```python
from build123d import *

# Parameters (mm, degrees)
BOSS_EXTRUDE1_DEPTH = 16
FILLET1_R           = 2
SKETCH2_W           = 15
SKETCH2_H           = 4.5
SKETCH2_H_2         = 6
SKETCH2_R           = 0.75
CUT_EXTRUDE1_DEPTH  = 32
SKETCH4_R           = 1.6
CUT_EXTRUDE2_DEPTH  = 92
CUT_EXTRUDE4_DEPTH  = 80.584099309
BOSS_EXTRUDE2_DEPTH = 3
DRAFT1_ANGLE        = 70
DRAFT2_START        = -8.5
DRAFT2_DEPTH        = 3
CUT_EXTRUDE5_DEPTH  = 0.5
FILLET4_R           = 0.5
FILLET3_R           = 2
CHAMFER1_SIZE       = 3


# Read off the part's stored shape, not the designer's step: Draft2
with BuildPart() as part:
    # Sketch1 → Boss-Extrude1 (new, symmetric)
    with BuildSketch(Plane(origin=(0, 0, 0), x_dir=(0, 0, -1), z_dir=(1, 0, 0))):
        Polygon((0, 16), (0, -17), (25.401923789, -60.997422612), (47.052558883, -48.497422612), (45.552558883, -45.899346401), (26.5, -56.899346401), (3, -16.196152423), (3, 16), align=None)
    extrude(amount=BOSS_EXTRUDE1_DEPTH, both=True)

    # Fillet1
    fillet1_edges = [part.edges().sort_by_distance(p)[0] for p in [
        (-16, 16, -1.5),
        (16, 16, -1.5),
    ]]
    fillet(fillet1_edges, radius=FILLET1_R)

    # Sketch2 → Cut-Extrude1 (cut)
    with BuildSketch(Plane(origin=(0, 0, -3), x_dir=(-1, 0, 0), z_dir=(0, 0, -1))):
        with Locations((0, 5.25)):
            Rectangle(SKETCH2_W, SKETCH2_H)
        Rectangle(SKETCH2_W, SKETCH2_H_2)
        with BuildLine():
            Line((-9, -3), (-7.5, -3))
            Line((-7.5, -3), (-7.5, 3))
            Line((-7.5, 3), (-9, 3))
            ThreePointArc((-9, 3), (-12, 0), (-9, -3))
        make_face()
        with Locations((0, -5.25)):
            Rectangle(SKETCH2_W, SKETCH2_H)
        with BuildLine():
            Line((7.5, 3), (7.5, -3))
            Line((7.5, -3), (9, -3))
            ThreePointArc((9, -3), (12, 0), (9, 3))
            Line((9, 3), (7.5, 3))
        make_face()
        with Locations((14, -14)):
            Circle(SKETCH2_R)
        with Locations((-14, -14)):
            Circle(SKETCH2_R)
        with Locations((-14, 14)):
            Circle(SKETCH2_R)
        with Locations((14, 14)):
            Circle(SKETCH2_R)
    extrude(amount=-CUT_EXTRUDE1_DEPTH, mode=Mode.SUBTRACT)

    # Sketch4 → Cut-Extrude2 (cut)
    with BuildSketch(Plane(origin=(0, -56.747422612, -32.763139721), x_dir=(1, 0, 0), z_dir=(0, -0.8660254037844379, -0.5000000000000014))):
        with Locations(Location((-4, -12.5, 0), (0, 0, 270))):
            Circle(SKETCH4_R)
        with Locations(Location((4, -12.5, 0), (0, 0, 270))):
            Circle(SKETCH4_R)
    extrude(amount=-CUT_EXTRUDE2_DEPTH, mode=Mode.SUBTRACT)

    # Sketch7 → Cut-Extrude4 (cut, symmetric)
    with BuildSketch(Plane(origin=(0, -2.75, 4.763139721), x_dir=(-1, 0, 0), z_dir=(0, 0.500000000000002, -0.8660254037844375))):
        Polygon((-10, -65.526279442), (-10, -26.526279442), (-16, -20.526279442), (-16, -65.526279442), align=None)
    cut_extrude4 = extrude(amount=CUT_EXTRUDE4_DEPTH, both=True, mode=Mode.SUBTRACT)

    # Sketch5 → Boss-Extrude2 (add)
    with BuildSketch(Plane(origin=(10, 0, 0), x_dir=(0, 0, -1), z_dir=(1, 0, 0))):
        Polygon((36.892304845, -50.899346401), (3, -11.196152423), (3, -16.196152423), (26.5, -56.899346401), align=None)
    boss_extrude2 = extrude(amount=-BOSS_EXTRUDE2_DEPTH)

    # Draft1
    draft1_faces = [part.faces().sort_by_distance(p)[0] for p in [
        (13, -23.874355653, -5.700961894),
    ]]
    draft(draft1_faces, Plane(origin=(16, 0, 0), x_dir=(0, 0, 1), z_dir=(1, 0, 0)), DRAFT1_ANGLE)

    # Mirror2: Cut-Extrude4, Boss-Extrude2 across plane
    add(cut_extrude4.mirror(Plane(origin=(0, 0, 0), x_dir=(0, 0, 1), z_dir=(1, 0, 0))), mode=Mode.SUBTRACT)
    add(boss_extrude2.mirror(Plane(origin=(0, 0, 0), x_dir=(0, 0, 1), z_dir=(1, 0, 0))))

    # Draft2 outline → Draft2 (add)
    with BuildSketch(Plane(origin=(0, 0, 0), x_dir=(1, 0, 0), z_dir=(0, 0.5000000000000018, -0.8660254037844377)).offset(DRAFT2_START)):
        Polygon((-10, 26.526279442), (-10, 37.011143958), (-16, 20.526279442), align=None)
    extrude(amount=DRAFT2_DEPTH)

    # Sketch8 → Cut-Extrude5 (cut)
    with BuildSketch(Plane.XY):
        with BuildLine():
            Line((3.75, -12.8), (11.25, -12.8))
            ThreePointArc((11.25, -12.8), (11.85, -13.4), (11.25, -14))
            Line((11.25, -14), (3.75, -14))
            ThreePointArc((3.75, -14), (3.15, -13.4), (3.75, -12.8))
        make_face()
    extrude(amount=-CUT_EXTRUDE5_DEPTH, mode=Mode.SUBTRACT)

    # Fillet4
    fillet4_edges = [part.edges().sort_by_distance(p)[0] for p in [
        (7.5, -12.8, -0.5),
        (11.85, -13.4, -0.5),
        (7.5, -14, -0.5),
        (3.15, -13.4, -0.5),
    ]]
    fillet(fillet4_edges, radius=FILLET4_R - 0.0001)  # a hair under: the kernel refuses the full size

    # Fillet3
    fillet3_edges = [part.edges().sort_by_distance(p)[0] for p in [
        (-7.5, 3, -1.5),
        (-7.5, -3, -1.5),
        (7.5, -3, -1.5),
        (7.5, 3, -1.5),
    ]]
    fillet(fillet3_edges, radius=FILLET3_R)

    # Chamfer1
    chamfer1_edges = [part.edges().sort_by_distance(p)[0] for p in [
        (10, -47.198384506, -46.302558883),
        (-10, -47.198384506, -46.302558883),
    ]]
    chamfer(chamfer1_edges, length=CHAMFER1_SIZE)


solid = part.part
```
Work out the finished part from the listing and answer in its coordinate system (mm). A direction names the side the tool comes from. Give positions to 0.01 mm unless a question says otherwise; leave off trailing zeros. Write each loop counter-clockwise with the first axis right and the second up, starting at its lowest first coordinate (ties: lowest second). Pieces come first, ordered by that corner, then holes.
(1) Which of the six approach directions +Z, -Z, +X, -X, +Y, -Y give full straight-line access (tool end or side, diameter ignored) to faces 1 (the flat face through (12.38, -23.56, -7.25)), 2 (the flat face through (16, -4, -1)), 3 (the flat face through (0.098, -36.833, -14.914)), 4 (the cylindrical face through (12, 0, -2)), 5 (the flat face through (0.14, -54.835, -36.076))?
Final values:
face 1: -Z, +X, +Y
face 2: +Z, -Z, +X, +Y, -Y
face 3: +Y
face 4: +Z, -Z
face 5: -Z, +X, -X, -Y
(2) The part is cut by section C-C on z = -15.5. Write down the section's boundary in (x, y).
Final values:
outline: (-10, -43.85) - (10, -43.85) - (10, -25.84) - (7, -25.84) - (7, -37.85) - (-7, -37.85) - (-7, -25.84) - (-10, -25.84) - close
(3) The part is cut by section A-A on y = -23. Write down the section's boundary in (x, z), plus the area to 3 significant figures.
Final values:
outline: (-15.59, -3.46) - (-14.96, -6.93) - (-10, -6.93) - (-10, -13.08) - (-7, -13.08) - (-7, -6.93) - (7, -6.93) - (7, -13.08) - (10, -13.08) - (10, -6.93) - (14.96, -6.93) - (15.59, -3.46) - close
area: 143 mm2
(4) The mould has two halves that part along Z. Classify faces 6 (the cylindrical face through (-12, 0, -2)), 7 (the flat face through (0.1, -51.3, -36.2)), 8 (the flat face through (-8.479, -47.956, -45.032)): pulls with the +Z half, pulls with the -Z half, needs draft (parallel to the pull), parting line crosses it, or undercut.
Final values:
face 6: needs draft
face 7: undercut
face 8: pulls with the -Z half
(5) Straight lines are drawn through the part: line 1 (X direction, y = -44.5, z = -26); line 2 (Y direction, x = -14, z = -2); line 3 (Y direction, x = -14, z = -1.8). For each, find the intervals that lie inside material, in ascending order.
Final values:
line 1: x = -10 to -7, 7 to 10
line 2: y = -20.46 to -14.75, -13.25 to 13.25, 14.75 to 16
line 3: y = -20.12 to -14.75, -13.25 to 13.25, 14.75 to 16
(6) The part is cut by section B-B on z = -35. Write down the section's boundary in (x, y).
Final values:
outline: (-10, -55.46) - (10, -55.46) - (10, -48.68) - (7, -48.68) - (7, -51.99) - (-7, -51.99) - (-7, -48.68) - (-10, -48.68) - close
(7) Flat-ended cylindrical pins translate along their axes: pin 1 Ø1.5 at (x, z) = (-1, -14.5) entering from +Y; pin 2 Ø1.2 at (x, y) = (-14, 14) entering from +Z; pin 3 Ø1.7 at (x, y) = (14, -14) entering from +Z; pin 4 Ø17 at (y, z) = (-29, -26.5) entering from -X. Find the tip coordinate at first contact, or state that the pin passes through.
Final values:
pin 1: stops at y = -34.82
pin 2: passes through
pin 3: stops at z = 0
pin 4: stops at x = -10
